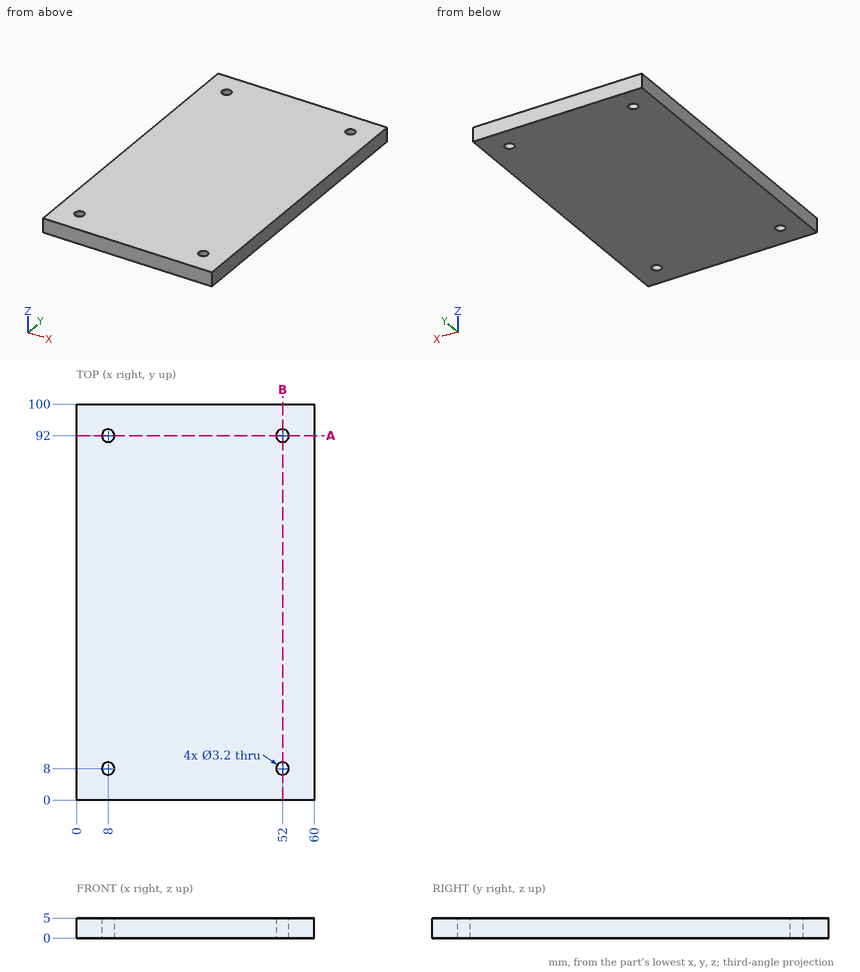
Study the drawing (mm; zero at the part's minimum x, y, z) and answer. Give positions to 0.01 mm unless a question says otherwise; leave off trailing zeros. Order: outer loops, then holes, each group sorted by start corner. A loop starts at its lowest first (then second) coordinate and runs counter-clockwise, first axis right, second up. Notation, with made-up numbers: M 84,-9 L 131,-9 A14 cw 131,12 Z; hole C 65,-12 d9. An arc over 180 degrees is marked long. Put each result on its own line as item: value. Start each with the question number.
Item 1: Flat-ended cylindrical pins translate along their axes: P1, Ø2.5, axis at x = 8, y = 8, coming from the -Z side; P2, Ø5, axis at x = 50, y = 51.5, coming from the -Z side. Find the tip coordinate at first contact, or state that the pin passes through.
Item 2: Find the intervals of material crossed by line 1 along Y through (x, z) = (52, 1.1); line 2 along X through (y, z) = (8, 3.95); line 3 along X through (y, z) = (7, 0.5), in increasing order.
Item 3: The part is cut by section A-A, the plane y = 92. Determine the outline of the cut face in (x, z), and give its area (3 significant figures).
Item 4: The part is cut by section B-B, the plane x = 52. Determine the outline of the cut face in (y, z), and give its area (3 significant figures).
Answer key:
1. P1: passes through
1. P2: stops at z = 0
2. line 1: y = 0 to 6.4, 9.6 to 90.4, 93.6 to 100
2. line 2: x = 0 to 6.4, 9.6 to 50.4, 53.6 to 60
2. line 3: x = 0 to 6.75, 9.25 to 50.75, 53.25 to 60
3. outline: M 0,0 L 6.4,0 L 6.4,5 L 0,5 Z; M 9.6,0 L 50.4,0 L 50.4,5 L 9.6,5 Z; M 53.6,0 L 60,0 L 60,5 L 53.6,5 Z
3. area: 268 mm²
4. outline: M 0,0 L 6.4,0 L 6.4,5 L 0,5 Z; M 9.6,0 L 90.4,0 L 90.4,5 L 9.6,5 Z; M 93.6,0 L 100,0 L 100,5 L 93.6,5 Z
4. area: 468 mm²
